Print and shaded views of the part. All mm, measured from the part's lowest x, y and z. A direction names the side the tool comes from. Give positions to 0.01 mm unless a question says otherwise; leave off trailing zeros. Order: outer loops, then holes, each group sorted by start corner. A loop starts at its lowest first (then second) coordinate and runs counter-clockwise, first axis right, second up. Notation, with made-up numbers: (56, 4.25) - (81, 4.25) arc R15 ccw to (81, 16.25) - close; hole circle Ø11 at (89, 19). An arc over 180 degrees is marked (long way). Answer in a Markdown table with one row per item.
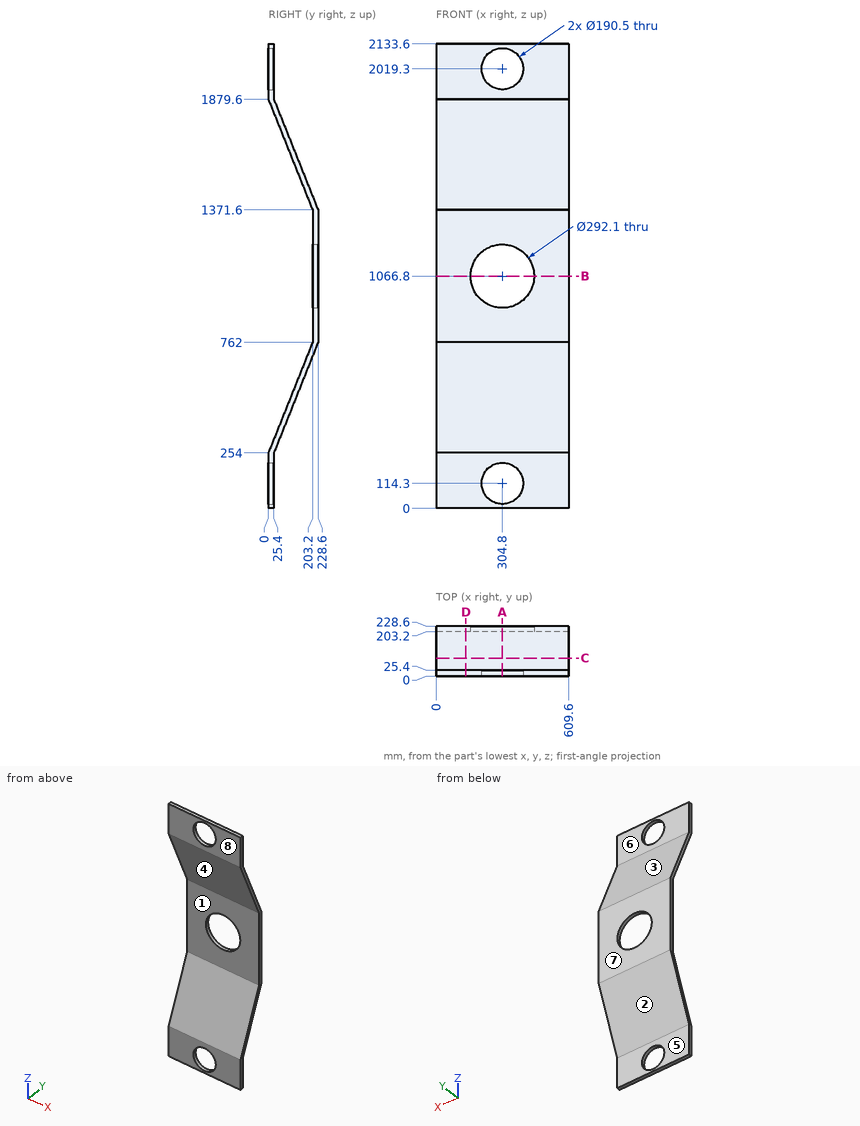
1. Cut at C-C on y = 82. Write the cut outline in (x, z), and give its area (3 significant figures).
Check result:
| item | result |
|---|---|
| outline | (0, 395.5) - (609.6, 395.5) - (609.6, 459) - (0, 459) - close; (0, 1674.6) - (609.6, 1674.6) - (609.6, 1738.1) - (0, 1738.1) - close |
| area | 77,400 mm² |
2. Probe line 1 (X direction, y = 6.5, z = 114.3); line 2 (X direction, y = 222, z = 1066.8); line 3 (Y direction, x = 233, z = 1955.5). List the from-to ranges inside material, lowest first.
Check result:
| item | result |
|---|---|
| line 1 | x = 0 to 209.55, 400.05 to 609.6 |
| line 2 | x = 0 to 158.75, 450.85 to 609.6 |
| line 3 | y = 0 to 25.4 |
3. Cut at A-A on x = 304.8. Write the cut outline in (y, z), and give its area (3 significant figures).
Check result:
| item | result |
|---|---|
| outline | (0, 0) - (25.4, 0) - (25.4, 19.05) - (0, 19.05) - close; (0, 209.55) - (25.4, 209.55) - (25.4, 254) - (228.6, 762) - (228.6, 920.75) - (203.2, 920.75) - (203.2, 762) - (0, 254) - close; (0, 1879.6) - (203.2, 1371.6) - (203.2, 1212.85) - (228.6, 1212.85) - (228.6, 1371.6) - (25.4, 1879.6) - (25.4, 1924.05) - (0, 1924.05) - close; (0, 2114.55) - (25.4, 2114.55) - (25.4, 2133.6) - (0, 2133.6) - close |
| area | 37,100 mm² |
4. Cut at D-D on x = 136.5. Write the cut outline in (y, z), and give its area (3 significant figures).
Check result:
| item | result |
|---|---|
| outline | (0, 0) - (25.4, 0) - (25.4, 254) - (228.6, 762) - (228.6, 1371.6) - (25.4, 1879.6) - (25.4, 2133.6) - (0, 2133.6) - (0, 1879.6) - (203.2, 1371.6) - (203.2, 762) - (0, 254) - close |
| area | 54,200 mm² |
5. Which spindle directions (+Z, -Z, +X, -X, +Y, -Y) get a long thin tool onto all of the face, cutting with end or side? Do the marked faces 4, 5, 6, 7 and 8. Say none if no direction does.
Check result:
| item | result |
|---|---|
| face 4 | +X, -X, -Y |
| face 5 | -Z, +X, -X, +Y |
| face 6 | +Z, +X, -X, +Y |
| face 7 | +Z, -Z, +X, -X, +Y |
| face 8 | +Z, -Z, +X, -X, -Y |
6. Two-plate mould, pull along Z, no slides. Class the marked faces 1, 2 and 3: +Z half, -Z half, draft (parallel to the pull), parting line (faces both ways), or undercut.
Check result:
| item | result |
|---|---|
| face 1 | undercut |
| face 2 | -Z half |
| face 3 | +Z half |
7. Cut at B-B on z = 1066.8. Write the cut outline in (x, y).
Check result:
| item | result |
|---|---|
| outline | (0, 203.2) - (158.75, 203.2) - (158.75, 228.6) - (0, 228.6) - close; (450.85, 203.2) - (609.6, 203.2) - (609.6, 228.6) - (450.85, 228.6) - close |
8. Drop flat-ended pins along their axis: P1, Ø12, axis at x = 472, z = 1429.5, coming from the +Y side; P2, Ø1, axis at x = 117, z = 1533.5, coming from the -Y side; P3, Ø5, axis at y = 194, z = 713, coming from the -X side. Give the stop position or say it passes through.
Check result:
| item | result |
|---|---|
| P1 | stops at y = 207.84 |
| P2 | stops at y = 138.24 |
| P3 | stops at x = 0 |
